from build123d import *

# Parameters (mm, degrees)
F0_W     = 50.3577142954
F0_H     = 47.1017286181
F1_DEPTH = 800
F2_DEPTH = 600
F3_DEPTH = 600
F4_T     = -18
F5_DEPTH = 80
F6_DEPTH = 25
F7_DEPTH = 80


with BuildPart() as f1:
    # F0 (on Top) → F1 (new body)
    with BuildSketch(Plane.XY):
        with Locations((25.1788571477, -23.5508643091)):
            Rectangle(F0_W, F0_H)
    extrude(amount=F1_DEPTH)

    # F2 (add): a face of the model
    f2_faces = [f1.faces().sort_by_distance(p)[0] for p in [
        (0, -23.5508643091, 400),
    ]]
    extrude(f2_faces, amount=-F2_DEPTH)

    # F3 (add): a face of the model
    f3_faces = [f1.faces().sort_by_distance(p)[0] for p in [
        (300, -47.1017286181, 400),
    ]]
    extrude(f3_faces, amount=-F3_DEPTH)

    # F4
    f4_openings = [f1.faces().sort_by_distance(p)[0] for p in [
        (300, 252.898271, 800),
        (300, -47.101729, 400),
    ]]
    offset(amount=F4_T, openings=f4_openings)

    # F5 (add): a face of the model
    f5_faces = [f1.faces().sort_by_distance(p)[0] for p in [
        (9, -38.6164472439, 800),
    ]]
    extrude(f5_faces, amount=F5_DEPTH)

    # F6 (cut): a face of the model
    f6_faces = [f1.faces().sort_by_distance(p)[0] for p in [
        (300, 534.8982713819, 449),
    ]]
    extrude(f6_faces, amount=-F6_DEPTH, mode=Mode.SUBTRACT)

    # F7 (cut): faces of the model
    f7_faces = [f1.faces().sort_by_distance(p)[0] for p in [
        (591, 252.8982713819, 880),
        (9, 252.8982713819, 880),
    ]]
    extrude(f7_faces, amount=-F7_DEPTH, mode=Mode.SUBTRACT)


solid = f1.part
Source: CAD feature listing. Evaluate the final solid. Frame: model axes, mm. A direction names the side the tool comes from. Give positions to 0.01 mm unless a question says otherwise; leave off trailing zeros. Write each loop counter-clockwise with the first axis right and the second up, starting at its lowest first coordinate (ties: lowest second). Pieces come first, ordered by that corner, then holes. Notation, with made-up numbers: M -40,57 L 13,57 A18 ccw 13,88 Z; hole C 5.25,66.5 d9. An arc over 180 degrees is marked long. Answer as a JSON object with one key per item and string values.
Q1. Mould query, pull axis X, two halves, no side actions, for faces 3 (the face through (296, 257, 0)), 4 (the face through (0, 249, 394)), 5 (the face through (18, 249, 404)). Classes: +X half, -X half, draft (parallel to the pull), parting line (faces both ways), or undercut.
Geometry check:
{"face 3": "draft", "face 4": "-X half", "face 5": "undercut"}
Q2. Cut plane A-A, the plane z = 434.5. Return the cut outline in (x, y), then the cut area to 3 significant figures.
Geometry check:
{"outline": "M 0,-47.1 L 18,-47.1 L 18,552.9 L 0,552.9 Z; M 582,-47.1 L 600,-47.1 L 600,552.9 L 582,552.9 Z", "area": "21,600 mm^2"}
Q3. Cut plane B-B, the plane y = 512. Return the cut outline in (x, z), then the cut area to 3 significant figures.
Geometry check:
{"outline": "M 0,0 L 600,0 L 600,800 L 582,800 L 582,18 L 18,18 L 18,800 L 0,800 Z", "area": "39,000 mm^2"}
Q4. Access query for faces 1 (the face through (600, 249, 394)), 2 (the face through (296, 257, 18)). Directions: +Z, -Z, +X, -X, +Y, -Y. A direction counts if a zero-diameter tool reaches every point of the face in a straight line with its end or side. Return the directions, or none.
Geometry check:
{"face 1": "+Z, -Z, +X, +Y, -Y", "face 2": "+Z, +Y, -Y"}
Q5. Ray query, line 1 along X through (y, z) = (421, 534.5); line 2 along Z through (x, y) = (495.5, -7). Return the intervals inside material, ascending.
Geometry check:
{"line 1": "x = 0 to 18, 582 to 600", "line 2": "z = 0 to 18"}
Q6. Cut plane C-C, the plane x = 201. Return the cut outline in (y, z), then the cut area to 3 significant figures.
Geometry check:
{"outline": "M -47.1,0 L 552.9,0 L 552.9,18 L -47.1,18 Z", "area": "10,800 mm^2"}
